Study the drawing (mm; zero at the part's minimum x, y, z) and answer. A direction names the side the tool comes from. Coordinates: 2 decimals unless noted, no trailing zeros. Loops run counter-clockwise (first coordinate to the right, second up) from the corner with the lowest first, then second, coordinate; pieces in that order, holes last. Notation, with made-up numbers: (47, 48.25) - (82, 48.25) arc R15 cw to (82, 52.25) - close; hole circle Ø11 at (41.5, 9.5). An arc over 180 degrees is marked (long way). Use CSV: the item, a comma, the result in double quotes.
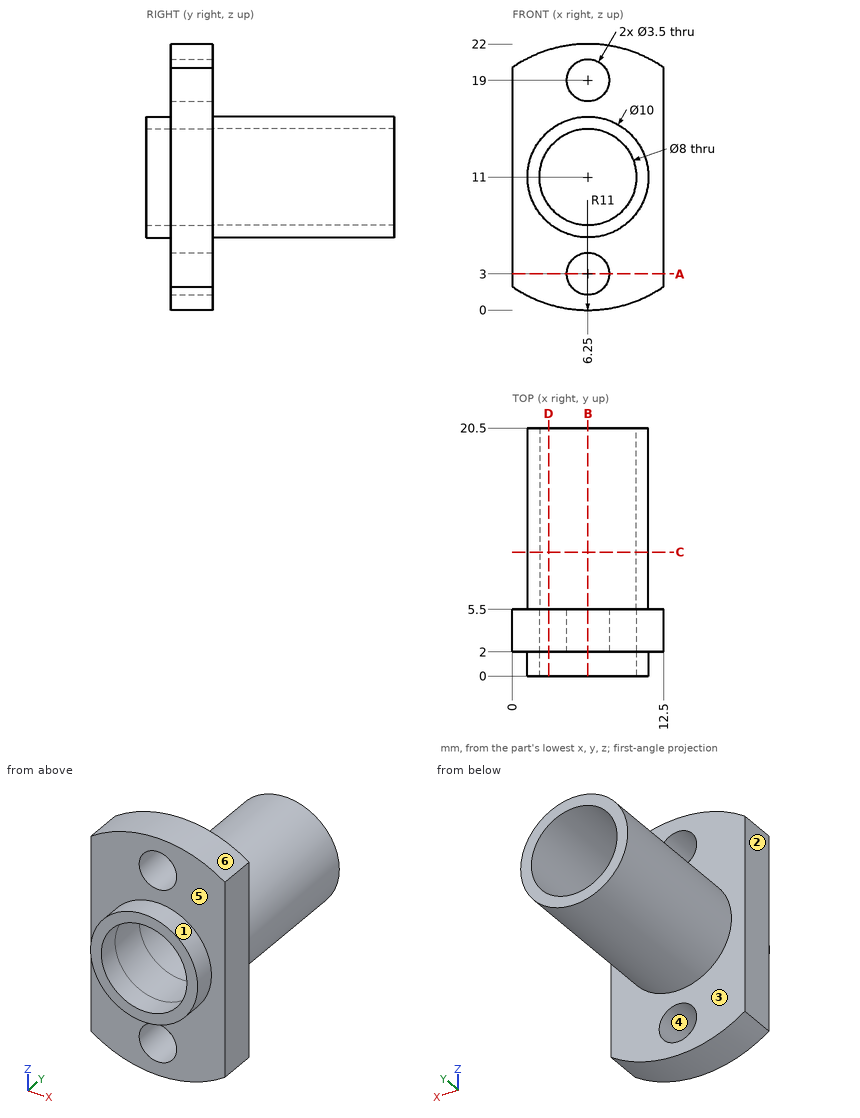
Q1. The part is cut by section C-C on y = 10.25. Determine the outline of the cut face in (x, z), and give its area (3 significant figures).
Reported:
outline,"circle Ø10 at (6.25, 11); hole circle Ø8 at (6.25, 11)"
area,"28.3 mm²"
Q2. Given P1, Ø3, axis at x = 6.25, z = 19, coming from the -Y side; P2, Ø8, axis at y = 15.5, z = 4, coming from the -X side; P3, Ø1, axis at x = 11, y = 13.5, coming from the +Z side; P4, Ø4, axis at x = 6.25, z = 3, coming from the +Y side, each flat-ended and moving along its own axis, determine where each tip first touches the part or whether it passes through.
Reported:
P1,"passes through"
P2,"stops at x = 2.25"
P3,"stops at z = 13.63"
P4,"stops at y = 5.5"
Q3. For a pull along Z with two mould halves and no side action, classify the marked faces 4, 5 and 6 as +Z half, -Z half, draft (parallel to the pull), parting line (faces both ways), or undercut.
Reported:
face 4,"undercut"
face 5,"draft"
face 6,"+Z half"
Q4. The part is cut by section B-B on x = 6.25. Determine the outline of the cut face in (y, z), and give its area (3 significant figures).
Reported:
outline,"(0, 6) - (2, 6) - (2, 4.75) - (5.5, 4.75) - (5.5, 6) - (20.5, 6) - (20.5, 7) - (0, 7) - close; (0, 15) - (20.5, 15) - (20.5, 16) - (5.5, 16) - (5.5, 17.25) - (2, 17.25) - (2, 16) - (0, 16) - close; (2, 0) - (5.5, 0) - (5.5, 1.25) - (2, 1.25) - close; (2, 20.75) - (5.5, 20.75) - (5.5, 22) - (2, 22) - close"
area,"58.5 mm²"
Q5. The part is cut by section D-D on x = 3. Determine the outline of the cut face in (y, z).
Reported:
outline,"(0, 7.2) - (2, 7.2) - (2, 0.49) - (5.5, 0.49) - (5.5, 7.2) - (20.5, 7.2) - (20.5, 8.67) - (0, 8.67) - close; (0, 13.33) - (20.5, 13.33) - (20.5, 14.8) - (5.5, 14.8) - (5.5, 21.51) - (2, 21.51) - (2, 14.8) - (0, 14.8) - close"
Q6. The part is cut by section A-A on z = 3. Determine the outline of the cut face in (x, y).
Reported:
outline,"(0, 2) - (4.5, 2) - (4.5, 5.5) - (0, 5.5) - close; (8, 2) - (12.5, 2) - (12.5, 5.5) - (8, 5.5) - close"
Q7. Find the intervals of material crossed by probe 1 along Z at (x, y) = (6.25, 3.15); probe 2 along X at (y, z) = (4.7, 19); probe 3 along X at (y, z) = (0.5, 11), in increasing order. Write a range as [from, to].
Reported:
probe 1,"z = [0, 1.25], [4.75, 7], [15, 17.25], [20.75, 22]"
probe 2,"x = [0, 4.5], [8, 12.5]"
probe 3,"x = [1.25, 2.25], [10.25, 11.25]"
Q8. A tool of negligible diameter and unlimited length cuts with its end or side. For the marked faces 1, 2 and 3, from which of +Z, -Z, +X, -X, +Y, -Y can it reach the whole face along a straight path? Write none if from no direction.
Reported:
face 1,"-Y"
face 2,"+Z, -Z, -X, +Y, -Y"
face 3,"+Y"
